Model file for the job. Use its own axes, mm. A direction names the side the tool comes from. Coordinates: 2 decimals unless noted, no trailing zeros. Write each loop counter-clockwise with the first axis right and the second up, starting at its lowest first coordinate (ties: lowest second). Pieces come first, ordered by that corner, then holes. Notation, with made-up numbers: M 78.5,-17.75 L 136.5,-17.75 A30 ccw 136.5,9.25 Z; hole C 48.25,55 d5. An arc over 180 degrees is marked long. One line per question, with ' | ' between items. Start each with the question number.
(1) Cut at C-C (x = 0). Write the cut outline in (y, z).
(2) Tool access for faces 4 (the face through (0, 13, 1)), 5 (the face through (0, 0, 0)), 6 (the face through (-2, 25, 0)): list every direction of +Z, -Z, +X, -X, +Y, -Y with a clear straight run to the whole face (end or side of a thin tool).
(3) Two-plate mould, pull along Z, no slides. Class faces 1 (the face through (-7.95, 19.35, 6.1)), 2 (the face through (8.52, 18.93, -2.68)), 3 (the face through (0, 26, 0)): +Z half, -Z half, draft (parallel to the pull), parting line (faces both ways), or undercut.
(4) Cut at B-B (y = 8.5). Write the cut outline in (x, z), plus the area to 3 significant figures.
(5) Cut at A-A (z = 0). Write the cut outline in (x, y).
(6) Flat gauge pins, fed straight in: pin 1 Ø12 at (x, z) = (8.5, -7.5) entering from -Y; pin 2 Ø1 at (y, z) = (22, 0.5) entering from -X; pin 3 Ø1 at (y, z) = (5, -2) entering from -X; pin 4 Ø6 at (y, z) = (21, -7.5) entering from +X. Where does each tip first touch, or does it go through?
(7) Wall check: probe 1 along Y at (x, z) = (-3.5, -2.75); probe 2 along Z at (x, y) = (-0.5, 24.75); probe 3 along X at (y, z) = (17, -5.5). Give the ranges that are in metal, low to high.
from build123d import *

# Parameters (mm, degrees)
SKETCH1_W = 1
SKETCH1_H = 25


with BuildPart() as part:
    # Sketch1 → Revolve1 (revolve)
    with BuildSketch(Plane.XY):
        with Locations((0.5, 12.5)):
            Rectangle(SKETCH1_W, SKETCH1_H)
    revolve(axis=Axis((0, 0, 0), (0, 1, 0)))

    # Sketch2 → Revolve2 (revolve)
    with BuildSketch(Plane.XY):
        Polygon((0, 25), (10, 25), (8.267349052, 15.173648178), (9.252156805, 15), (11.191753593, 26), (0, 26), align=None)
    revolve(axis=Axis((0, 0, 0), (0, 1, 0)))


solid = part.part
Filled in:
1) outline: M 0,-1 L 25,-1 L 25,-10 L 15.17,-8.27 L 15,-9.25 L 26,-11.19 L 26,11.19 L 15,9.25 L 15.17,8.27 L 25,10 L 25,1 L 0,1 Z
2) face 4: -Y | face 5: +Z, -Z, +X, -X, -Y | face 6: none
3) face 1: parting line | face 2: undercut | face 3: draft
4) outline: C 0,0 d2 | area: 3.14 mm²
5) outline: M -11.19,26 L -9.25,15 L -8.27,15.17 L -10,25 L -1,25 L -1,0 L 1,0 L 1,25 L 10,25 L 8.27,15.17 L 9.25,15 L 11.19,26 Z
6) pin 1: y = 15 | pin 2: x = -10.57 | pin 3: through | pin 4: x = 9.39
7) probe 1: 25 to 26 | probe 2: -10.96 to -9.94, -0.87 to 0.87, 9.94 to 10.96 | probe 3: -7.87 to -6.6, 6.6 to 7.87
